Geometry: final body of the model. Coordinates: model frame, mm. Round coordinates to 2 decimals unless told otherwise and drop trailing zeros. Order: outer loops, then holes, each group sorted by start corner. A loop starts at its lowest first (then second) coordinate and runs counter-clockwise, first axis right, second up. Notation, with made-up numbers: M -12,-35.75 L -6,-35.75 A27 ccw -6,-12.75 Z; hole C 82.25,60.5 d8. An arc over 180 degrees is marked long. Put each result on its own line as item: value. Start each with the question number.
1) Section A-A, the plane x = 30. Return loops of the section in (y, z).
2) Section C-C, the plane y = -25. Count the separate pieces of the cut face and the enclosed holes in it, then the cut area to 3 significant figures.
3) Section D-D, the plane x = -5.5. Return loops of the section in (y, z), then the cut area to 4 significant figures.
4) First-contact query: P1, Ø5.5, axis at x = 30, z = -2.5, coming from the -Y side; P2, Ø1.5, axis at y = 1, z = -3.5, coming from the +X side; P3, Ø10, axis at x = -9, y = -21, coming from the -Z side. Flat tips, straight axial feed; report the tip coordinate or a pass-through.
5) Section B-B, the plane x = 50. Return loops of the section in (y, z).
6) Material intervals for probe 1 along Y at (x, z) = (27, -1.75); probe 2 along Z at (x, y) = (-4.5, -39), sorted ascending. Write a range as [from, to].
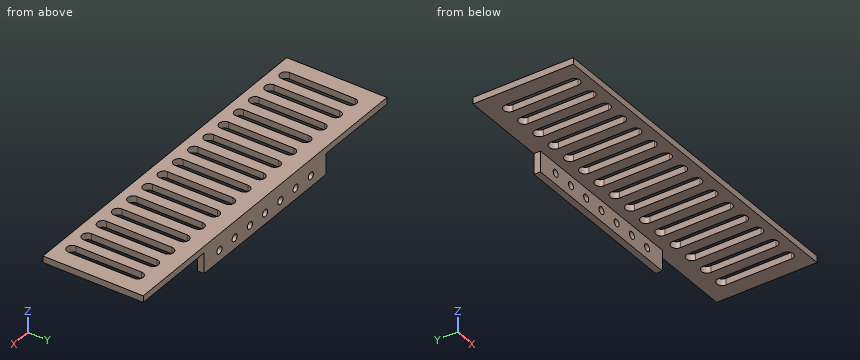
from build123d import *

# Parameters (mm, degrees)
SKETCH_1_W          = 80
SKETCH_1_H          = 15
EXTRUDE_1_DEPTH     = 3
SKETCH_2_R          = 1.65
CUT_EXTRUDE_1_DEPTH = 3
SKETCH_3_W          = 80
SKETCH_3_H          = 3
EXTRUDE_2_DEPTH     = 43
SKETCH_4_W          = 3
SKETCH_4_H          = 46
EXTRUDE_3_DEPTH     = 40
SKETCH_5_W          = 3
SKETCH_5_H          = 46
EXTRUDE_4_DEPTH     = 40
SKETCH_8_W          = 2.5
SKETCH_8_H          = 3
CUT_EXTRUDE_3_DEPTH = 80
CUT_EXTRUDE_4_DEPTH = 80


with BuildPart() as part:
    # 草图1 → 凸台-拉伸1 (new body)
    with BuildSketch(Plane(origin=(0, 0, 0), x_dir=(1, 0, 0), z_dir=(0, 1, 0))):
        Rectangle(SKETCH_1_W, SKETCH_1_H)
    extrude(amount=EXTRUDE_1_DEPTH)

    # 草图2 → 切除-拉伸1 (cut)
    with BuildSketch(Plane(origin=(0, 3, 0), x_dir=(1, 0, 0), z_dir=(0, 1, 0))):
        with Locations(Location((-30, 2.5, 0), (0, 0, 270))):
            Circle(SKETCH_2_R)
        with Locations(Location((-20, 2.5, 0), (0, 0, 270))):
            Circle(SKETCH_2_R)
        with Locations(Location((-10, 2.5, 0), (0, 0, 270))):
            Circle(SKETCH_2_R)
        with Locations(Location((0, 2.5, 0), (0, 0, 270))):
            Circle(SKETCH_2_R)
        with Locations(Location((10, 2.5, 0), (0, 0, 270))):
            Circle(SKETCH_2_R)
        with Locations(Location((20, 2.5, 0), (0, 0, 270))):
            Circle(SKETCH_2_R)
        with Locations(Location((30, 2.5, 0), (0, 0, 270))):
            Circle(SKETCH_2_R)
    extrude(amount=-CUT_EXTRUDE_1_DEPTH, mode=Mode.SUBTRACT)

    # 草图3 → 凸台-拉伸2 (add)
    with BuildSketch(Plane.XZ):
        with Locations((0, 3.5)):
            Rectangle(SKETCH_3_W, SKETCH_3_H)
    extrude(amount=EXTRUDE_2_DEPTH)

    # 草图4 → 凸台-拉伸3 (add)
    with BuildSketch(Plane(origin=(40, 0, 0), x_dir=(0, 0, -1), z_dir=(1, 0, 0))):
        with Locations((-3.5, -20)):
            Rectangle(SKETCH_4_W, SKETCH_4_H)
    extrude(amount=EXTRUDE_3_DEPTH)

    # 草图5 → 凸台-拉伸4 (add)
    with BuildSketch(Plane.ZY.offset(40)):
        with Locations((3.5, -20)):
            Rectangle(SKETCH_5_W, SKETCH_5_H)
    extrude(amount=EXTRUDE_4_DEPTH)

    # 草图8 → 切除-拉伸3 (cut)
    with BuildSketch(Plane.ZY.offset(40)):
        with Locations((6.25, 1.5)):
            Rectangle(SKETCH_8_W, SKETCH_8_H)
    extrude(amount=-CUT_EXTRUDE_3_DEPTH, mode=Mode.SUBTRACT)

    # 草图9 → 切除-拉伸4 (cut)
    with BuildSketch(Plane(origin=(0, 0, 2), x_dir=(-1, 0, 0), z_dir=(0, 0, -1))):
        with BuildLine():
            Line((-67.5, -6.520841628), (-67.5, -36.520841628))
            ThreePointArc((-67.5, -36.520841628), (-70, -39.020841628), (-72.5, -36.520841628))
            Line((-72.5, -36.520841628), (-72.5, -6.520841628))
            ThreePointArc((-72.5, -6.520841628), (-70, -4.020841628), (-67.5, -6.520841628))
        make_face()
        with BuildLine():
            Line((-57.5, -6.520841628), (-57.5, -36.520841628))
            ThreePointArc((-57.5, -36.520841628), (-60, -39.020841628), (-62.5, -36.520841628))
            Line((-62.5, -36.520841628), (-62.5, -6.520841628))
            ThreePointArc((-62.5, -6.520841628), (-60, -4.020841628), (-57.5, -6.520841628))
        make_face()
        with BuildLine():
            Line((-47.5, -6.520841628), (-47.5, -36.520841628))
            ThreePointArc((-47.5, -36.520841628), (-50, -39.020841628), (-52.5, -36.520841628))
            Line((-52.5, -36.520841628), (-52.5, -6.520841628))
            ThreePointArc((-52.5, -6.520841628), (-50, -4.020841628), (-47.5, -6.520841628))
        make_face()
        with BuildLine():
            Line((-37.5, -6.520841628), (-37.5, -36.520841628))
            ThreePointArc((-37.5, -36.520841628), (-40, -39.020841628), (-42.5, -36.520841628))
            Line((-42.5, -36.520841628), (-42.5, -6.520841628))
            ThreePointArc((-42.5, -6.520841628), (-40, -4.020841628), (-37.5, -6.520841628))
        make_face()
        with BuildLine():
            Line((-27.5, -6.520841628), (-27.5, -36.520841628))
            ThreePointArc((-27.5, -36.520841628), (-30, -39.020841628), (-32.5, -36.520841628))
            Line((-32.5, -36.520841628), (-32.5, -6.520841628))
            ThreePointArc((-32.5, -6.520841628), (-30, -4.020841628), (-27.5, -6.520841628))
        make_face()
        with BuildLine():
            Line((-17.5, -6.520841628), (-17.5, -36.520841628))
            ThreePointArc((-17.5, -36.520841628), (-20, -39.020841628), (-22.5, -36.520841628))
            Line((-22.5, -36.520841628), (-22.5, -6.520841628))
            ThreePointArc((-22.5, -6.520841628), (-20, -4.020841628), (-17.5, -6.520841628))
        make_face()
        with BuildLine():
            Line((-7.5, -6.520841628), (-7.5, -36.520841628))
            ThreePointArc((-7.5, -36.520841628), (-10, -39.020841628), (-12.5, -36.520841628))
            Line((-12.5, -36.520841628), (-12.5, -6.520841628))
            ThreePointArc((-12.5, -6.520841628), (-10, -4.020841628), (-7.5, -6.520841628))
        make_face()
        with BuildLine():
            Line((2.5, -6.520841628), (2.5, -36.520841628))
            ThreePointArc((2.5, -36.520841628), (0, -39.020841628), (-2.5, -36.520841628))
            Line((-2.5, -36.520841628), (-2.5, -6.520841628))
            ThreePointArc((-2.5, -6.520841628), (0, -4.020841628), (2.5, -6.520841628))
        make_face()
        with BuildLine():
            Line((12.5, -6.520841628), (12.5, -36.520841628))
            ThreePointArc((12.5, -36.520841628), (10, -39.020841628), (7.5, -36.520841628))
            Line((7.5, -36.520841628), (7.5, -6.520841628))
            ThreePointArc((7.5, -6.520841628), (10, -4.020841628), (12.5, -6.520841628))
        make_face()
        with BuildLine():
            Line((22.5, -6.520841628), (22.5, -36.520841628))
            ThreePointArc((22.5, -36.520841628), (20, -39.020841628), (17.5, -36.520841628))
            Line((17.5, -36.520841628), (17.5, -6.520841628))
            ThreePointArc((17.5, -6.520841628), (20, -4.020841628), (22.5, -6.520841628))
        make_face()
        with BuildLine():
            Line((32.5, -6.520841628), (32.5, -36.520841628))
            ThreePointArc((32.5, -36.520841628), (30, -39.020841628), (27.5, -36.520841628))
            Line((27.5, -36.520841628), (27.5, -6.520841628))
            ThreePointArc((27.5, -6.520841628), (30, -4.020841628), (32.5, -6.520841628))
        make_face()
        with BuildLine():
            Line((42.5, -6.520841628), (42.5, -36.520841628))
            ThreePointArc((42.5, -36.520841628), (40, -39.020841628), (37.5, -36.520841628))
            Line((37.5, -36.520841628), (37.5, -6.520841628))
            ThreePointArc((37.5, -6.520841628), (40, -4.020841628), (42.5, -6.520841628))
        make_face()
        with BuildLine():
            Line((52.5, -6.520841628), (52.5, -36.520841628))
            ThreePointArc((52.5, -36.520841628), (50, -39.020841628), (47.5, -36.520841628))
            Line((47.5, -36.520841628), (47.5, -6.520841628))
            ThreePointArc((47.5, -6.520841628), (50, -4.020841628), (52.5, -6.520841628))
        make_face()
        with BuildLine():
            Line((62.5, -6.520841628), (62.5, -36.520841628))
            ThreePointArc((62.5, -36.520841628), (60, -39.020841628), (57.5, -36.520841628))
            Line((57.5, -36.520841628), (57.5, -6.520841628))
            ThreePointArc((57.5, -6.520841628), (60, -4.020841628), (62.5, -6.520841628))
        make_face()
        with BuildLine():
            Line((72.5, -6.520841628), (72.5, -36.520841628))
            ThreePointArc((72.5, -36.520841628), (70, -39.020841628), (67.5, -36.520841628))
            Line((67.5, -36.520841628), (67.5, -6.520841628))
            ThreePointArc((67.5, -6.520841628), (70, -4.020841628), (72.5, -6.520841628))
        make_face()
    extrude(amount=-CUT_EXTRUDE_4_DEPTH, mode=Mode.SUBTRACT)


solid = part.part
Result sheet:
1. outline: M -43,2 L -39.02,2 L -39.02,5 L -43,5 Z; M -4.02,2 L 0,2 L 0,-0.85 L 3,-0.85 L 3,5 L -4.02,5 Z; M 0,-7.5 L 3,-7.5 L 3,-4.15 L 0,-4.15 Z
2. separate pieces: 16
2. enclosed holes: 0
2. area: 255 mm2
3. outline: M -43,2 L 0,2 L 0,-7.5 L 3,-7.5 L 3,5 L -43,5 Z
3. area: 166.5 mm2
4. P1: stops at y = 0
4. P2: stops at x = 40
4. P3: stops at z = 2
5. outline: M -43,2 L -39.02,2 L -39.02,5 L -43,5 Z; M -4.02,2 L 3,2 L 3,5 L -4.02,5 Z
6. probe 1: y = [0, 3]
6. probe 2: z = [2, 5]
